Input: part model. Units: mm. Frame: model coordinates. A direction names the side the tool comes from. Round coordinates to 2 decimals unless told otherwise and drop trailing zeros. Order: outer loops, then holes, each group sorted by start corner. A loop starts at its lowest first (then second) coordinate and runs counter-clockwise, first axis right, second up. Notation, with made-up numbers: M 71.25,24 L 124.25,24 A28 ccw 124.25,58 Z; hole C -27.75,-0.5 d3. An arc over 180 degrees is marked long. One line per question, with ' | ' between items.
```python
from build123d import *

# Parameters (mm, degrees)
F1_R = 11
F3_T = -0.8


with BuildPart() as f2:
    # F2: sweep along a path in F0
    with BuildLine(Plane.XZ) as f2_path:
        Line((0, 0), (0, 400))
        ThreePointArc((0, 400), (-4.3933982822, 410.6066017178), (-15, 415))
        Line((-15, 415), (-55, 415))
        ThreePointArc((-55, 415), (-63.419035512, 413.3253497152), (-70.5563491861, 408.5563491861))
        Line((-70.5563491861, 408.5563491861), (-91.7695526217, 387.3431457505))
    # F1 (on Top) → F2 (sweep)
    with BuildSketch(Plane.XY):
        Circle(F1_R)
    sweep(path=f2_path.line)

    # F3
    f3_openings = [f2.faces().sort_by_distance(p)[0] for p in [
        (-91.769553, 0, 387.343146),
        (0, 0, 0),
    ]]
    offset(amount=F3_T, openings=f3_openings)


solid = f2.part
```
Item 1: Section query A-A, the plane y = 3.5. Return loops of the section in (x, z), plus the area to 3 significant figures.
Report:
outline: M -99.14,394.72 L -98.54,394.12 L -77.33,415.33 A31.58 cw -55,424.58 L -15,424.58 A24.58 cw 9.58,400 L 9.58,0 L 10.43,0 L 10.43,400 A25.43 ccw -15,425.43 L -55,425.43 A32.43 ccw -77.93,415.93 Z; M -84.99,380.57 L -84.4,379.97 L -63.18,401.18 A11.57 cw -55,404.57 L -15,404.57 A4.57 cw -10.43,400 L -10.43,0 L -9.58,0 L -9.58,400 A5.42 ccw -15,405.42 L -55,405.42 A12.42 ccw -63.78,401.78 Z | area: 866 mm²
Item 2: Section query C-C, the plane x = -37.5. Return loops of the section in (y, z), plus the area to 3 significant figures.
Report:
outline: C 0,415 d22; hole C 0,415 d20.4 | area: 53.3 mm²
Item 3: Mould query, pull axis Y, two halves, no side actions, for faces 4 (the flat face through (-86.044, 6.467, 381.618)), 5 (the cylindrical face through (-88.73, 3.3, 405.22)), 6 (the cylindrical face through (4.707, -9.049, 202.8)), 7 (the cylindrical face through (-74.1, 0.4, 390.6)). Classes: +Y half, -Y half, draft (parallel to the pull), parting line (faces both ways), or undercut.
Report:
face 4: draft | face 5: parting line | face 6: undercut | face 7: undercut
Item 4: Line query: line 1 along X through (y, z) = (-1.25, 64); line 2 along Y through (x, z) = (-32, 415); line 3 along Z through (x, y) = (-14.5, -0.75). Output: solid intervals per line, ascending. Write a range as from..to.
Report:
line 1: -10.93..-10.12, 10.12..10.93 | line 2: -11..-10.2, 10.2..11 | line 3: 403.99..404.8, 425.17..425.97
Item 5: Section query D-D, the plane z = 387. Give the number of separate pieces and of enclosed holes in the cut face, plus the area to 3 significant figures.
Report:
separate pieces: 2 | enclosed holes: 1 | area: 89.9 mm²
Item 6: Section query B-B, the plane z = 301. Return loops of the section in (x, y).
Report:
outline: C 0,0 d22; hole C 0,0 d20.4
Item 7: Access query for faces 1 (the flat face through (3, -10, 0)), 2 (the cylindrical face through (-35, 0, 404)), 3 (the cylindrical face through (-2.38, -10.74, 202.8)). Directions: +Z, -Z, +X, -X, +Y, -Y. A direction counts if a zero-diameter tool reaches every point of the face in a straight line with its end or side. Return the directions, or none.
Report:
face 1: -Z, +X, -X, +Y, -Y | face 2: none | face 3: -Z
Item 8: First-contact query: pin 1 (12 mm diameter, centred on x = 0, y = 0, fed in from +Z); pin 2 (2 mm diameter, centred on y = 5.5, z = 55.5, fed in from +X); pin 3 (8 mm diameter, centred on x = -76.5, y = -4, fed in from +Z). Flat tips, straight axial feed; report the tip coordinate or a pass-through.
Report:
pin 1: z = 424.39 | pin 2: x = 10.04 | pin 3: z = 420.45
